```python
from build123d import *

# Parameters (mm, degrees)
SKETCH1_W           = 50.8
SKETCH1_H           = 55.9562
BOSS_EXTRUDE1_DEPTH = 10.16
SKETCH2_W           = 50.8
SKETCH2_H           = 3.8608
CUT_EXTRUDE1_DEPTH  = 2.032
CUT_EXTRUDE2_DEPTH  = 51.8
SKETCH4_R           = 3.175
CUT_EXTRUDE3_DEPTH  = 11.16
SKETCH5_W           = 50.8
SKETCH5_H           = 33.9852
CUT_EXTRUDE4_DEPTH  = 4.064
CUT_EXTRUDE5_DEPTH  = 4.064
CUT_EXTRUDE6_DEPTH  = 4.064


with BuildPart() as part:
    # Sketch1 → Boss-Extrude1 (new body)
    with BuildSketch(Plane.XY):
        Rectangle(SKETCH1_W, SKETCH1_H)
    extrude(amount=BOSS_EXTRUDE1_DEPTH)

    # Sketch2 → Cut-Extrude1 (cut)
    with BuildSketch(Plane.XY.offset(10.16)):
        with Locations((0, 26.0477)):
            Rectangle(SKETCH2_W, SKETCH2_H)
        with Locations((0, -26.0477)):
            Rectangle(SKETCH2_W, SKETCH2_H)
    extrude(amount=-CUT_EXTRUDE1_DEPTH, mode=Mode.SUBTRACT)

    # Sketch3 → Cut-Extrude2 (cut, through all)
    with BuildSketch(Plane.ZY.offset(25.4)):
        Polygon((8.128, 24.1173), (1.440898242, 27.9781), (8.128, 27.9781), align=None)
        Polygon((8.128, -24.1173), (1.440898242, -27.9781), (8.128, -27.9781), align=None)
    extrude(amount=-CUT_EXTRUDE2_DEPTH, mode=Mode.SUBTRACT)

    # Sketch4 → Cut-Extrude3 (cut, through all)
    with BuildSketch(Plane.XY.offset(10.16)):
        Circle(SKETCH4_R)
    extrude(amount=-CUT_EXTRUDE3_DEPTH, mode=Mode.SUBTRACT)

    # Sketch5 → Cut-Extrude4 (cut)
    with BuildSketch(Plane(origin=(0, 0, 0), x_dir=(-1, 0, 0), z_dir=(0, 0, -1))):
        Rectangle(SKETCH5_W, SKETCH5_H)
    extrude(amount=-CUT_EXTRUDE4_DEPTH, mode=Mode.SUBTRACT)

    # Sketch6 → Cut-Extrude5 (cut)
    with BuildSketch(Plane(origin=(0, 0, 0), x_dir=(-1, 0, 0), z_dir=(0, 0, -1))):
        with BuildLine():
            Line((6.35, 21.0058), (-6.35, 21.0058))
            ThreePointArc((-6.35, 21.0058), (-8.59506403, 20.07586403), (-9.525, 17.8308))
            Line((-9.525, 17.8308), (-9.525, -17.8308))
            ThreePointArc((-9.525, -17.8308), (-8.59506403, -20.07586403), (-6.35, -21.0058))
            Line((-6.35, -21.0058), (6.35, -21.0058))
            ThreePointArc((6.35, -21.0058), (8.59506403, -20.07586403), (9.525, -17.8308))
            Line((9.525, -17.8308), (9.525, 17.8308))
            ThreePointArc((9.525, 17.8308), (8.59506403, 20.07586403), (6.35, 21.0058))
        make_face()
    extrude(amount=-CUT_EXTRUDE5_DEPTH, mode=Mode.SUBTRACT)

    # Sketch7 → Cut-Extrude6 (cut)
    with BuildSketch(Plane(origin=(0, 0, 0), x_dir=(-1, 0, 0), z_dir=(0, 0, -1))):
        Polygon((-12.7, 16.9926), (-25.4, 20.658774209), (-25.4, 16.9926), align=None)
        Polygon((-12.861684204, -16.9926), (-25.4, -20.6121), (-25.4, -16.9926), align=None)
        Polygon((12.7, -16.9926), (25.4, -20.658774209), (25.4, -16.9926), align=None)
        Polygon((12.7, 16.9926), (25.4, 20.658774209), (25.4, 16.9926), align=None)
    extrude(amount=-CUT_EXTRUDE6_DEPTH, mode=Mode.SUBTRACT)


solid = part.part
```
The model under review builds one solid part; all positions refer to its coordinate system, in mm. A direction names the side the tool comes from. Round coordinates to 2 decimals unless told otherwise and drop trailing zeros. Write each loop counter-clockwise with the first axis right and the second up, starting at its lowest first coordinate (ties: lowest second). Pieces come first, ordered by that corner, then holes.
(1) Wall thickness on L1, parallel to Y at x = -12.5, z = 0.75; L2, parallel to Y at x = 0, z = 8.25 (3 decimals); L3, parallel to Z at x = 1, y = 7.5: over which ranges is each line inside the solid? List them lowest first.
(2) Machinability: for faces 1 (the flat face through (-18.96, 18.8, 2)), 2 (the flat face through (-11, 16.993, 2)), 3 (the cylindrical face through (8.57, 20.1, 2)), 4 (the flat face through (0, 24.117, 9)), which of the approach directions +Z, -Z, +X, -X, +Y, -Y give a long, thin tool a straight path to every point of the face, cutting with its end or side? Answer none if there is none.
(3) We need section B-B on x = 0. Give the boundary of the cut face in (y, z) (3 decimals).
(4) We need section C-C on z = 9.5. Give the boundary of the cut face in (x, y) (3 decimals), and give its area (3 significant figures).
(5) Mouldability with a two-part tool opening along X and no side actions: class faces 5 (the flat face through (0, -27.978, 1)), 6 (the flat face through (-18.96, -18.8, 2)), 7 (the cylindrical face through (-8.62, 20.05, 2)) as +X half, -X half, draft (parallel to the pull), parting line (faces both ways), or undercut.
(6) We need section A-A on y = 0. Give the boundary of the cut face in (x, z) (3 decimals).
(7) We need section D-D on x = -11. Give the boundary of the cut face in (y, z), and give its area (3 significant figures).
(8) Insertion check: pin 1 (10 mm diameter, centred on x = 0, y = 0, fed in from -Z); pin 2 (0.6 mm diameter, centred on x = 2, z = 8.5, fed in from -Y); pin 3 (1.6 mm diameter, centred on x = 12, z = 8.5, fed in from +Y). Each pin has a flat end and moves straight along its axis. Give the tip position at first contact, or say it passes through.
Findings below:
1. L1: y = -27.98 to -16.99, 16.99 to 27.98
1. L2: y = -24.117 to -3.175, 3.175 to 24.117
1. L3: z = 4.06 to 10.16
2. face 1: -Z, -X
2. face 2: -Z, +X, -X
2. face 3: -Z
2. face 4: +Z, +X, -X, +Y
3. outline: (-27.978, 0) - (-21.006, 0) - (-21.006, 4.064) - (-3.175, 4.064) - (-3.175, 10.16) - (-24.117, 10.16) - (-24.117, 8.128) - (-27.978, 1.441) - close; (3.175, 4.064) - (21.006, 4.064) - (21.006, 0) - (27.978, 0) - (27.978, 1.441) - (24.117, 8.128) - (24.117, 10.16) - (3.175, 10.16) - close
4. outline: (-25.4, -24.117) - (25.4, -24.117) - (25.4, 24.117) - (-25.4, 24.117) - close; hole circle Ø6.35 at (0, 0)
4. area: 2,420 mm2
5. face 5: draft
5. face 6: -X half
5. face 7: undercut
6. outline: (-25.4, 4.064) - (-3.175, 4.064) - (-3.175, 10.16) - (-25.4, 10.16) - close; (3.175, 4.064) - (25.4, 4.064) - (25.4, 10.16) - (3.175, 10.16) - close
7. outline: (-27.98, 0) - (-16.99, 0) - (-16.99, 4.06) - (16.99, 4.06) - (16.99, 0) - (27.98, 0) - (27.98, 1.44) - (24.12, 8.13) - (24.12, 10.16) - (-24.12, 10.16) - (-24.12, 8.13) - (-27.98, 1.44) - close
7. area: 389 mm2
8. pin 1: stops at z = 4.06
8. pin 2: stops at y = -24.12
8. pin 3: stops at y = 24.36
